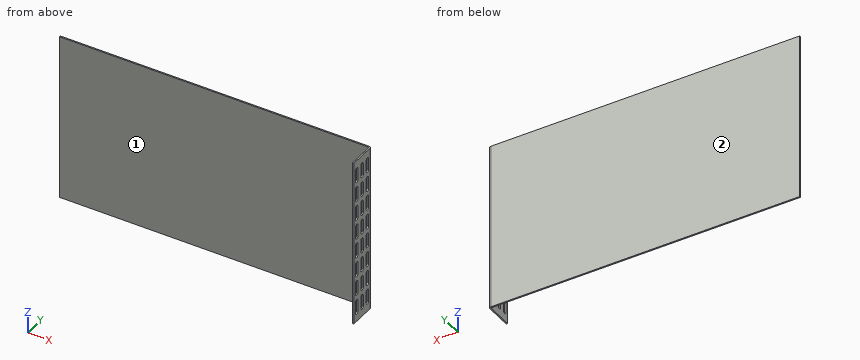
from build123d import *

# Parameters (mm, degrees)
BOSS_EXTRUDE1_DEPTH  = 60.198
FILLET1_R            = 0.4826
FILLET2_R            = 1.4732
CUT_EXTRUDE1_DEPTH   = 0.9906
LPATTERN1_COUNT      = 3
LPATTERN1_PITCH      = 6.1722
LPATTERN1_COUNT_DIR2 = 8
LPATTERN1_PITCH_DIR2 = 14.097


with BuildPart() as part:
    # Sketch1 → Boss-Extrude1 (new body, symmetric)
    with BuildSketch(Plane.XY):
        Polygon((0, 0), (0, 20.32), (-223.04375, 20.32), (-223.04375, 19.3294), (-0.9906, 19.3294), (-0.9906, 0), align=None)
    extrude(amount=BOSS_EXTRUDE1_DEPTH, both=True)

    # Fillet1
    fillet1_edges = [part.edges().sort_by_distance(p)[0] for p in [
        (-0.9906, 19.3294, 0),
    ]]
    fillet(fillet1_edges, radius=FILLET1_R)

    # Fillet2
    fillet2_edges = [part.edges().sort_by_distance(p)[0] for p in [
        (0, 20.32, 0),
    ]]
    fillet(fillet2_edges, radius=FILLET2_R)

    # Sketch2 → Cut-Extrude1 (cut)
    with BuildSketch(Plane(origin=(0, 0, 0), x_dir=(0, 0, -1), z_dir=(1, 0, 0))):
        with BuildLine():
            Line((-53.3908, 4.8514), (-45.3644, 4.8514))
            ThreePointArc((-45.3644, 4.8514), (-43.8912, 3.3782), (-45.3644, 1.905))
            Line((-45.3644, 1.905), (-53.3908, 1.905))
            ThreePointArc((-53.3908, 1.905), (-54.864, 3.3782), (-53.3908, 4.8514))
        make_face()
    cut_extrude1 = extrude(amount=-CUT_EXTRUDE1_DEPTH, mode=Mode.SUBTRACT)

    # LPattern1: Cut-Extrude1 3 × 8
    with Locations(*[(0, i * LPATTERN1_PITCH, -j * LPATTERN1_PITCH_DIR2) for i in range(LPATTERN1_COUNT) for j in range(LPATTERN1_COUNT_DIR2) if (i, j) != (0, 0)]):
        add(cut_extrude1, mode=Mode.SUBTRACT)


solid = part.part
Build history of the part. All positions in model axes, mm. Face numbers are marked on the shaded views. A direction names the side the tool comes from. Round coordinates to 2 decimals unless told otherwise and drop trailing zeros. Loops run counter-clockwise (first coordinate to the right, second up) from the corner with the lowest first, then second, coordinate; pieces in that order, holes last. Notation, with made-up numbers: (46, 81.25) -> (68, 81.25) arc R14 cw to (68, 88.25) -> close; hole circle Ø1 at (-12, 9.5). An arc over 180 degrees is marked (long way). Use CSV: the item, a comma, the result in double quotes. Start each with the question number.
Q1. Flat gauge pins, fed straight in: pin 1 Ø1 at (x, z) = (-122, -4) entering from -Y; pin 2 Ø1.1 at (x, z) = (-0.5, 7.5) entering from +Y; pin 3 Ø0.5 at (x, z) = (-0.5, 19.5) entering from +Y. Where does each tip first touch, or does it go through?
Q2. Saw through at B-B on x = -185. Give the cut face in (y, z).
Q3. Saw through at A-A on z = -36.5. Give the cut face in (x, y) (3 decimals), and give its area (3 significant figures).
Q4. Drill centre lines: L1, parallel to Y at x = -89, z = 14; L2, parallel to X at y = 13.5, z = 44. Where is each one in solid material? Low to high.
Q5. Which spindle directions (+Z, -Z, +X, -X, +Y, -Y) get a long thin tool onto all of the face, cutting with end or side? Do the marked faces 1 and 2. Say none if no direction does.
Solutions:
1,pin 1,"stops at y = 19.33"
1,pin 2,"stops at y = 20.26"
1,pin 3,"stops at y = 20.13"
2,outline,"(19.33, -60.2) -> (20.32, -60.2) -> (20.32, 60.2) -> (19.33, 60.2) -> close"
3,outline,"(-223.044, 19.329) -> (-1.473, 19.329) arc R0.483 cw to (-0.991, 18.847) -> (-0.991, 17.196) -> (0, 17.196) -> (0, 18.847) arc R1.473 ccw to (-1.473, 20.32) -> (-223.044, 20.32) -> close; (-0.991, 0) -> (0, 0) -> (0, 1.905) -> (-0.991, 1.905) -> close; (-0.991, 4.851) -> (0, 4.851) -> (0, 8.077) -> (-0.991, 8.077) -> close; (-0.991, 11.024) -> (0, 11.024) -> (0, 14.249) -> (-0.991, 14.249) -> close"
3,area,"231 mm^2"
4,L1,"y = 19.33 to 20.32"
4,L2,"x = -0.99 to 0"
5,face 1,"+Z, -Z, -X, -Y"
5,face 2,"+Z, -Z, +X, -X, +Y"
